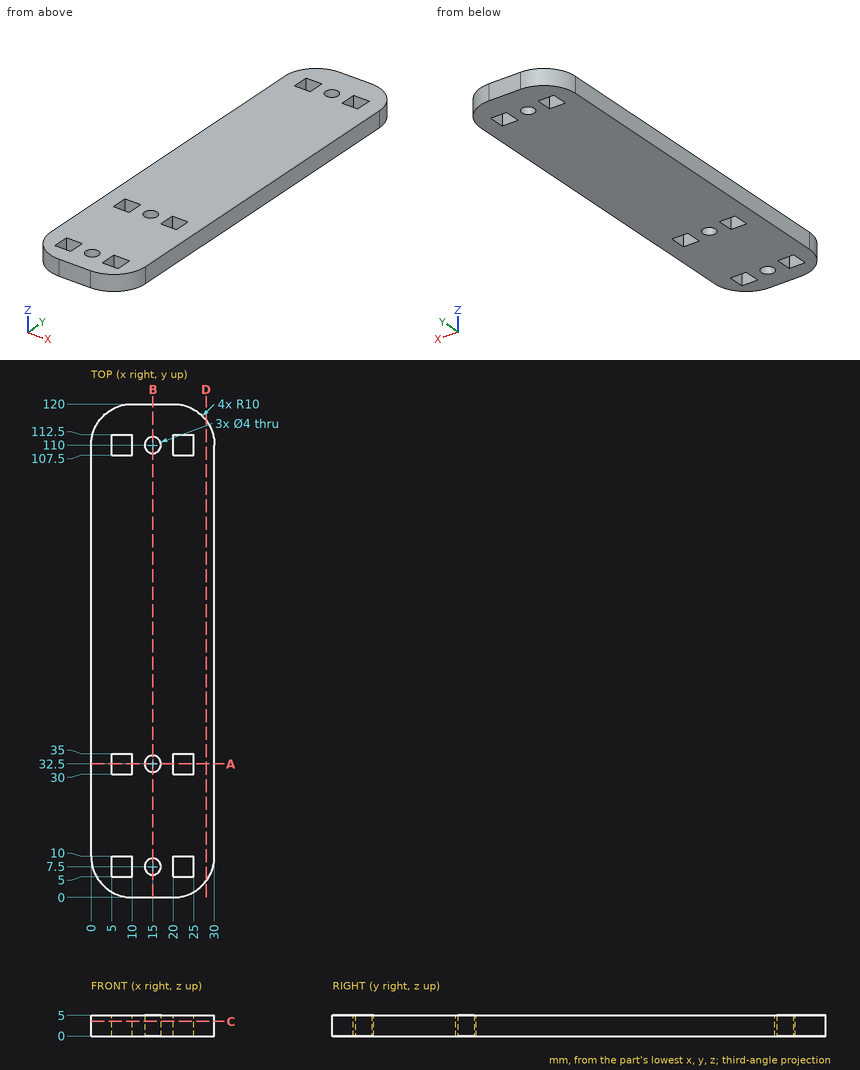
Geometry check sheet. Reference: drawing and pictorial views, mm from the part's lowest x, y, z. Coordinates: 2 decimals unless noted, no trailing zeros. Loops run counter-clockwise (first coordinate to the right, second up) from the corner with the lowest first, then second, coordinate; pieces in that order, holes last. Notation, with made-up numbers: (50, 8) -> (96, 8) arc R21 ccw to (96, 41) -> close; hole circle Ø11 at (49, -12.75). An arc over 180 degrees is marked (long way). Put each result on its own line as item: value.
1) Cross-section at B-B on x = 15. Record the boundary of the cut face in (y, z), plus the area to 3 significant figures.
Result set:
outline: (0, 0) -> (5.5, 0) -> (5.5, 5) -> (0, 5) -> close; (9.5, 0) -> (30.5, 0) -> (30.5, 5) -> (9.5, 5) -> close; (34.5, 0) -> (108, 0) -> (108, 5) -> (34.5, 5) -> close; (112, 0) -> (120, 0) -> (120, 5) -> (112, 5) -> close
area: 540 mm^2
2) Cross-section at C-C on z = 3.55. Count the separate pieces of the cut face and the enclosed holes in it, plus the area to 3 significant figures.
Result set:
separate pieces: 1
enclosed holes: 9
area: 3,330 mm^2
3) Cross-section at A-A on y = 32.5. Record the boundary of the cut face in (x, z).
Result set:
outline: (0, 0) -> (5, 0) -> (5, 5) -> (0, 5) -> close; (10, 0) -> (13, 0) -> (13, 5) -> (10, 5) -> close; (17, 0) -> (20, 0) -> (20, 5) -> (17, 5) -> close; (25, 0) -> (30, 0) -> (30, 5) -> (25, 5) -> close
4) Cross-section at D-D on x = 28. Record the boundary of the cut face in (y, z).
Result set:
outline: (4, 0) -> (116, 0) -> (116, 5) -> (4, 5) -> close
5) Gauge pin test, flat ends, axial feed: pin 1 Ø2.5 at (x, z) = (8, 2) entering from +Y; pin 2 Ø2.5 at (x, z) = (22.5, 3) entering from -Y; pin 3 Ø1.5 at (x, z) = (22, 4.5) entering from +Y. Record the tip position at first contact, or that the pin passes through.
Result set:
pin 1: stops at y = 119.97
pin 2: stops at y = 0.08
pin 3: stops at y = 119.92
6) Thickness scan on line 1 (Y direction, x = 9.75, z = 0.75); line 2 (Y direction, x = 15, z = 2); line 3 (X direction, y = 7, z = 2.15). Record the ranges inside material, lowest first.
Result set:
line 1: y = 0 to 5, 10 to 30, 35 to 107.5, 112.5 to 120
line 2: y = 0 to 5.5, 9.5 to 30.5, 34.5 to 108, 112 to 120
line 3: x = 0.46 to 5, 10 to 13.06, 16.94 to 20, 25 to 29.54
